Build history of the part. All positions in model axes, mm. Round coordinates to 2 decimals unless told otherwise and drop trailing zeros. Write each loop counter-clockwise with the first axis right and the second up, starting at its lowest first coordinate (ties: lowest second). Pieces come first, ordered by that corner, then holes.
1) Saw through at B-B (x = 23). Write the cut outline in (y, z).
2) Saw through at A-A (z = 0). Write the cut outline in (x, y), plus the area to 3 significant figures.
3) Saw through at C-C (x = -16.5). Write the cut outline in (y, z), plus the area to 3 significant figures.
4) Flat gauge pins, fed straight in: pin 1 (2 mm diameter, centred on x = -48.5, z = -23, fed in from +Y); pin 2 (3 mm diameter, centred on y = 4.5, z = 32, fed in from +X). Where does each tip first touch, or does it go through?
5) Saw through at D-D (x = 43.5). Write the cut outline in (y, z).
6) Wall check: probe 1 along X at (y, z) = (4.75, 0); probe 2 along X at (y, z) = (4.75, -22); probe 3 along X at (y, z) = (2.5, -40). Give the ranges that are in metal, low to high.
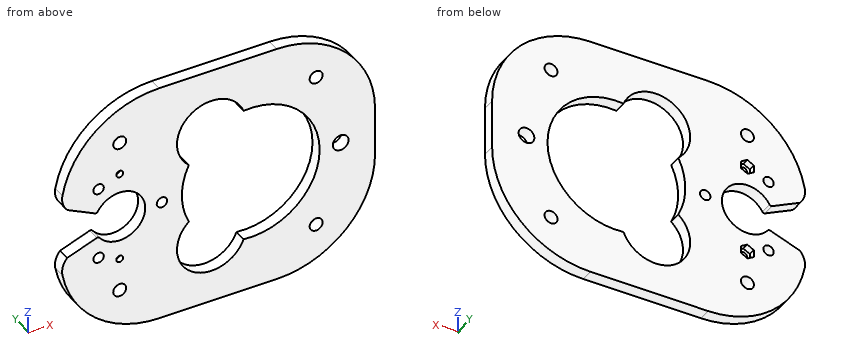
from build123d import *

# Parameters (mm, degrees)
SKETCH2_R                = 13
SKETCH2_R_2              = 4
BOSS_EXTRUDE1_DEPTH      = 6.35
FILLET1_R                = 50
M6_CLEARANCE_HOLE1_D     = 6.6
M6_CLEARANCE_HOLE1_DEPTH = 15
M6_CLEARANCE_HOLE1_TIP   = 1.982840043
FILLET2_R                = 10
CUT_EXTRUDE1_REACH       = 103.718
SKETCH5_R                = 2.65
SKETCH5_R_2              = 1.75
CUT_EXTRUDE2_DEPTH       = 3.5
CUT_EXTRUDE3_REACH       = 103.718
FILLET3_R                = 1
CUT_EXTRUDE4_REACH       = 103.718


with BuildPart() as part:
    # Sketch2 → Boss-Extrude1 (new body)
    with BuildSketch(Plane(origin=(0, 0, 0), x_dir=(1, 0, 0), z_dir=(0, 1, 0))):
        with BuildLine():
            ThreePointArc((-76.703745056, 13), (-79.7, 0), (-76.703745056, -13))
            Line((-76.703745056, -13), (-80, -13))
            Line((-80, -13), (-80, -62.5))
            Line((-80, -62.5), (80, -62.5))
            Line((80, -62.5), (80, 62.5))
            Line((80, 62.5), (-80, 62.5))
            Line((-80, 62.5), (-80, 13))
            Line((-80, 13), (-76.703745056, 13))
        make_face()
        with Locations(Location((-50, 0, 0), (0, 0, 270))):
            Circle(SKETCH2_R, mode=Mode.SUBTRACT)
        with Locations(Location((62.5, 0, 0), (0, 0, 270))):
            Circle(SKETCH2_R_2, mode=Mode.SUBTRACT)
    extrude(amount=BOSS_EXTRUDE1_DEPTH)

    # Fillet1
    # the kernel refuses this fillet: 50 mm, written as the material it takes off along each edge
    with BuildSketch(Plane(origin=(80, -125, 62.5), x_dir=(-1, 0, 0), z_dir=(0, 1, 0)), Plane(origin=(80, -125, -62.5), x_dir=(0, 0, 1), z_dir=(0, 1, 0))) as fillet1_piece_1:
        with BuildLine():
            CenterArc((FILLET1_R, -FILLET1_R), FILLET1_R, 90, 90)
            Line((0, -FILLET1_R), (-FILLET1_R * 0.02, -FILLET1_R))
            Line((-FILLET1_R * 0.02, -FILLET1_R), (-FILLET1_R * 0.02, FILLET1_R * 0.02))
            Line((-FILLET1_R * 0.02, FILLET1_R * 0.02), (FILLET1_R, FILLET1_R * 0.02))
            Line((FILLET1_R, FILLET1_R * 0.02), (FILLET1_R, 0))
        make_face()
    extrude(amount=256.35, mode=Mode.SUBTRACT)
    with BuildSketch(Plane(origin=(-80, -124.993749844, -62.5), x_dir=(1, 0, 0), z_dir=(0, 1, 0))) as fillet1_piece_2:
        with BuildLine():
            CenterArc((49.997499938, -50), FILLET1_R, 90, 89.427032655)
            Line((0, -49.5), (-0.999949999, -49.49))
            ThreePointArc((-0.999949999, -49.49), (-1, -24.75), (-1, 0))
            Line((-1, 0), (0, 1))
            Line((0, 1), (49.997499938, 1))
            Line((49.997499938, 1), (49.997499938, 0))
        make_face()
    extrude(amount=256.337499688, mode=Mode.SUBTRACT)
    with BuildSketch(Plane(origin=(-80, -124.993749844, 62.5), x_dir=(0, 0, -1), z_dir=(0, 1, 0))) as fillet1_piece_3:
        with BuildLine():
            CenterArc((50, -49.997499937), FILLET1_R, 90.572967345, 89.427032655)
            Line((0, -49.997499938), (-1, -49.997499938))
            Line((-1, -49.997499938), (-1, 0))
            Line((-1, 0), (0, 1))
            ThreePointArc((0, 1), (24.75, 1), (49.49, 0.999949999))
            Line((49.49, 0.999949999), (49.5, 0))
        make_face()
    extrude(amount=256.337499688, mode=Mode.SUBTRACT)

    # M6 Clearance Hole1
    with Locations(Plane(origin=(0, 6.35, 0), x_dir=(1, 0, 0), z_dir=(0, 1, 0))):
        with Locations((50, 40), (-50, -40), (-50, 40), (50, -40)):
            Hole(M6_CLEARANCE_HOLE1_D / 2, depth=M6_CLEARANCE_HOLE1_DEPTH)
            with Locations((0, 0, -(M6_CLEARANCE_HOLE1_DEPTH + M6_CLEARANCE_HOLE1_TIP / 2))):  # 118° drill point
                Cone(0, M6_CLEARANCE_HOLE1_D / 2, M6_CLEARANCE_HOLE1_TIP, mode=Mode.SUBTRACT)

    # Fillet2
    # the kernel refuses this fillet: 10 mm, written as the material it takes off along each edge
    with BuildSketch(Plane(origin=(-80, -21.546986926, 13), x_dir=(1, 0, 0), z_dir=(0, 1, 0))) as fillet2_piece_1:
        with BuildLine():
            CenterArc((10.662433046, -6.7630925), FILLET2_R, 137.444096304, 53.017550986)
            Line((0.828666324, -8.578865625), (0.631990989, -8.615181088))
            ThreePointArc((0.631990989, -8.615181088), (0.030066454, -4.326550643), (-0.19999, -0.002))
            Line((-0.19999, -0.002), (0, 0.2))
            ThreePointArc((0, 0.2), (1.648127472, 0.2), (3.148931382, 0.13526185))
            Line((3.148931382, 0.13526185), (3.296254944, 0))
        make_face()
    extrude(amount=49.443973852, mode=Mode.SUBTRACT)
    with BuildSketch(Plane(origin=(-80, -21.546986926, -13), x_dir=(1, 0, 0), z_dir=(0, 1, 0))) as fillet2_piece_2:
        with BuildLine():
            CenterArc((10.662433046, 6.7630925), FILLET2_R, 169.538352709, 53.017550986)
            Line((0.828666324, 8.578865625), (0.631990989, 8.615181088))
            ThreePointArc((0.631990989, 8.615181088), (0.030066454, 4.326550643), (-0.19999, 0.002))
            Line((-0.19999, 0.002), (0, -0.2))
            ThreePointArc((0, -0.2), (1.648127472, -0.2), (3.148931382, -0.13526185))
            Line((3.148931382, -0.13526185), (3.296254944, 0))
        make_face()
    extrude(amount=49.443973852, mode=Mode.SUBTRACT)

    # Sketch5 → Cut-Extrude1 (cut, up to next)
    with BuildSketch(Plane(origin=(0, 6.35, 0), x_dir=(1, 0, 0), z_dir=(0, 1, 0)), mode=Mode.PRIVATE) as cut_extrude1_sk1:
        with Locations(Location((-28.5, 0, 0), (0, 0, 270))):
            Circle(SKETCH5_R)
    cut_extrude1_tool1 = extrude(cut_extrude1_sk1.sketch, amount=-CUT_EXTRUDE1_REACH, mode=Mode.PRIVATE) & part.part
    # Sketch5 → Cut-Extrude1 (cut, up to next)
    with BuildSketch(Plane(origin=(0, 6.35, 0), x_dir=(1, 0, 0), z_dir=(0, 1, 0)), mode=Mode.PRIVATE) as cut_extrude1_sk2:
        with Locations(Location((-60.75, -18.619546181, 0), (0, 0, 270))):
            Circle(SKETCH5_R)
    cut_extrude1_tool2 = extrude(cut_extrude1_sk2.sketch, amount=-CUT_EXTRUDE1_REACH, mode=Mode.PRIVATE) & part.part
    # Sketch5 → Cut-Extrude1 (cut, up to next)
    with BuildSketch(Plane(origin=(0, 6.35, 0), x_dir=(1, 0, 0), z_dir=(0, 1, 0)), mode=Mode.PRIVATE) as cut_extrude1_sk3:
        with Locations(Location((-60.75, 18.619546181, 0), (0, 0, 270))):
            Circle(SKETCH5_R)
    cut_extrude1_tool3 = extrude(cut_extrude1_sk3.sketch, amount=-CUT_EXTRUDE1_REACH, mode=Mode.PRIVATE) & part.part
    # Sketch5 → Cut-Extrude1 (cut, up to next)
    with BuildSketch(Plane(origin=(0, 6.35, 0), x_dir=(1, 0, 0), z_dir=(0, 1, 0)), mode=Mode.PRIVATE) as cut_extrude1_sk4:
        with Locations(Location((-50, 23.015, 0), (0, 0, 270))):
            Circle(SKETCH5_R_2)
    cut_extrude1_tool4 = extrude(cut_extrude1_sk4.sketch, amount=-CUT_EXTRUDE1_REACH, mode=Mode.PRIVATE) & part.part
    # Sketch5 → Cut-Extrude1 (cut, up to next)
    with BuildSketch(Plane(origin=(0, 6.35, 0), x_dir=(1, 0, 0), z_dir=(0, 1, 0)), mode=Mode.PRIVATE) as cut_extrude1_sk5:
        with Locations(Location((-50, -23.015, 0), (0, 0, 270))):
            Circle(SKETCH5_R_2)
    cut_extrude1_tool5 = extrude(cut_extrude1_sk5.sketch, amount=-CUT_EXTRUDE1_REACH, mode=Mode.PRIVATE) & part.part
    add(cut_extrude1_tool1.solids().sort_by_distance((-28.5, 6.35, 0))[0], mode=Mode.SUBTRACT)
    add(cut_extrude1_tool2.solids().sort_by_distance((-60.75, 6.35, 18.619546))[0], mode=Mode.SUBTRACT)
    add(cut_extrude1_tool3.solids().sort_by_distance((-60.75, 6.35, -18.619546))[0], mode=Mode.SUBTRACT)
    add(cut_extrude1_tool4.solids().sort_by_distance((-50, 6.35, -23.015))[0], mode=Mode.SUBTRACT)
    add(cut_extrude1_tool5.solids().sort_by_distance((-50, 6.35, 23.015))[0], mode=Mode.SUBTRACT)

    # Sketch6 → Cut-Extrude2 (cut)
    with BuildSketch(Plane(origin=(0, 6.35, 0), x_dir=(1, 0, 0), z_dir=(0, 1, 0))):
        Polygon((-53.220697552, -24.941250403), (-49.942166993, -26.767331099), (-46.721469441, -24.841080696), (-46.779302448, -21.088749597), (-50.057833007, -19.262668901), (-53.278530559, -21.188919304), align=None)
        Polygon((-46.779302448, 24.941250403), (-50.057833007, 26.767331099), (-53.278530559, 24.841080696), (-53.220697552, 21.088749597), (-49.942166993, 19.262668901), (-46.721469441, 21.188919304), align=None)
    extrude(amount=-CUT_EXTRUDE2_DEPTH, mode=Mode.SUBTRACT)

    # Sketch7 → Cut-Extrude3 (cut, up to next)
    with BuildSketch(Plane(origin=(0, 6.35, 0), x_dir=(1, 0, 0), z_dir=(0, 1, 0)), mode=Mode.PRIVATE) as cut_extrude3_sk1:
        with BuildLine():
            Line((-76.703745056, 13), (-60.823662152, 7.200578978))
            ThreePointArc((-60.823662152, 7.200578978), (-62.970841385, 0.870214783), (-61.688507937, -5.69023569))
            Line((-61.688507937, -5.69023569), (-76.703745056, -13))
            ThreePointArc((-76.703745056, -13), (-79.7, 0), (-76.703745056, 13))
        make_face()
    cut_extrude3_tool1 = extrude(cut_extrude3_sk1.sketch, amount=-CUT_EXTRUDE3_REACH, mode=Mode.PRIVATE) & part.part
    add(cut_extrude3_tool1.solids().sort_by_distance((-71.4533, 6.35, -0.3701))[0], mode=Mode.SUBTRACT)

    # Fillet3
    fillet3_edges = [part.edges().sort_by_distance(p)[0] for p in [
        (-60.823662152, 3.175, -7.200578978),
        (-61.688507937, 3.175, 5.69023569),
    ]]
    fillet(fillet3_edges, radius=FILLET3_R)

    # Sketch8 → Cut-Extrude4 (cut, up to next)
    with BuildSketch(Plane(origin=(0, 6.35, 0), x_dir=(1, 0, 0), z_dir=(0, 1, 0)), mode=Mode.PRIVATE) as cut_extrude4_sk1:
        with BuildLine():
            ThreePointArc((13.086188506, -34.897759169), (51.803145873, 0), (13.086188506, 34.897759169))
            ThreePointArc((13.086188506, 34.897759169), (-13.347108623, 43.021646829), (-14.805555972, 15.406620499))
            ThreePointArc((-14.805555972, 15.406620499), (-18.369113715, 0), (-14.805555972, -15.406620499))
            ThreePointArc((-14.805555972, -15.406620499), (-13.347108623, -43.021646829), (13.086188506, -34.897759169))
        make_face()
    cut_extrude4_tool1 = extrude(cut_extrude4_sk1.sketch, amount=-CUT_EXTRUDE4_REACH, mode=Mode.PRIVATE) & part.part
    add(cut_extrude4_tool1.solids().sort_by_distance((11.588613, 6.35, 0))[0], mode=Mode.SUBTRACT)


solid = part.part
Evaluation:
1. outline: (0, -62.5) - (6.35, -62.5) - (6.35, -34.52) - (0, -34.52) - close; (0, 34.52) - (6.35, 34.52) - (6.35, 62.5) - (0, 62.5) - close
2. outline: (-37, 0) - (-31.15, 0) - (-31.15, 6.35) - (-37, 6.35) - close; (-25.85, 0) - (-18.37, 0) - (-18.37, 6.35) - (-25.85, 6.35) - close; (51.8, 0) - (58.5, 0) - (58.5, 6.35) - (51.8, 6.35) - close; (66.5, 0) - (80, 0) - (80, 6.35) - (66.5, 6.35) - close
2. area: 213 mm2
3. outline: (0, -62.5) - (6.35, -62.5) - (6.35, -40.19) - (0, -40.19) - close; (0, -17.1) - (6.35, -17.1) - (6.35, -11.3) - (0, -11.3) - close; (0, 11.3) - (6.35, 11.3) - (6.35, 17.1) - (0, 17.1) - close; (0, 40.19) - (6.35, 40.19) - (6.35, 62.5) - (0, 62.5) - close
3. area: 357 mm2
4. pin 1: stops at y = 2.85
4. pin 2: stops at x = 76.65
5. outline: (0, -60.64) - (6.35, -60.64) - (6.35, -22.67) - (0, -22.67) - close; (0, 22.67) - (6.35, 22.67) - (6.35, 60.64) - (0, 60.64) - close
6. probe 1: x = -37 to -31.15, -25.85 to -18.37, 51.8 to 58.5, 66.5 to 80
6. probe 2: x = -79.09 to -53.23, -46.73 to -19.53, 44.05 to 79.09
6. probe 3: x = -71.76 to -53.3, -46.7 to -16.67, 10.07 to 46.7, 53.3 to 71.76
